```python
from build123d import *

# Parameters (mm, degrees)
BOSS_EXTRU_3_DEPTH = 50
ESQUISSE3_W        = 80
ESQUISSE3_H        = 10
BOSS_EXTRU_4_DEPTH = 50
ESQUISSE4_R        = 15
ESQUISSE4_R_2      = 12
BOSS_EXTRU_5_DEPTH = 5
CONG_1_R           = 2
BOSS_EXTRU_6_DEPTH = 25
BOSS_EXTRU_7_DEPTH = 10


with BuildPart() as part:
    # Esquisse2 → Boss.-Extru.3 (new body)
    with BuildSketch(Plane.XY):
        Polygon((0, 0), (100, 0), (90, 10), (10, 10), align=None)
    extrude(amount=BOSS_EXTRU_3_DEPTH)

    # Esquisse3 → Boss.-Extru.4 (add)
    with BuildSketch(Plane.XY.offset(50)):
        with Locations((50, 15)):
            Rectangle(ESQUISSE3_W, ESQUISSE3_H)
    extrude(amount=-BOSS_EXTRU_4_DEPTH)

    # Esquisse4 → Boss.-Extru.5 (add)
    with BuildSketch(Plane(origin=(0, 20, 0), x_dir=(1, 0, 0), z_dir=(0, 1, 0))):
        with Locations((65, -25)):
            Circle(ESQUISSE4_R)
        with Locations((65, -25)):
            Circle(ESQUISSE4_R_2, mode=Mode.SUBTRACT)
    extrude(amount=BOSS_EXTRU_5_DEPTH)

    # Congé1
    cong_1_edges = [part.edges().sort_by_distance(p)[0] for p in [
        (50, 20, 25),
    ]]
    fillet(cong_1_edges, radius=CONG_1_R)

    # Esquisse5 → Boss.-Extru.6 (add)
    with BuildSketch(Plane(origin=(0, 20, 0), x_dir=(1, 0, 0), z_dir=(0, 1, 0))):
        Polygon((20, 0), (10, 0), (10, -50), (20, -50), (20, -10), (50, -10), (50, 0), align=None)
    extrude(amount=BOSS_EXTRU_6_DEPTH)

    # Esquisse6 → Boss.-Extru.7 (add)
    with BuildSketch(Plane.XY.offset(50)):
        Polygon((20, 45), (50, 20), (20, 20), align=None)
    extrude(amount=-BOSS_EXTRU_7_DEPTH)


solid = part.part
```
Source: CAD feature listing. Evaluate the final solid. Frame: model axes, mm. A direction names the side the tool comes from. Coordinates: 2 decimals unless noted, no trailing zeros. Write each loop counter-clockwise with the first axis right and the second up, starting at its lowest first coordinate (ties: lowest second). Pieces come first, ordered by that corner, then holes. Notation, with made-up numbers: (-35.75, 21) -> (10.25, 21) arc R26 ccw to (10.25, 43) -> close; hole circle Ø2 at (83, 65.5). An arc over 180 degrees is marked (long way). Return JSON: item names as keys, results as strings. Group by question number.
1) Contact query for flat-ended pins moving along their axis: P1, Ø3, axis at y = 16.5, z = 24, coming from the +X side; P2, Ø1.5, axis at y = 17, z = 14.5, coming from the -X side; P3, Ø12, axis at y = 13, z = 12.5, coming from the -X side. Output: stop coordinate, or through.
2) Section query D-D, the plane y = 28.5. Return loops of the section in (x, z).
3) Section query B-B, the plane x = 65. Return loops of the section in (y, z), plus the area to 3 significant figures.
4) Ray query, line 1 along X through (y, z) = (23.65, 25); line 2 along Z through (x, y) = (65, 22); line 3 along Z through (x, y) = (42.5, 32.5). Return the intervals inside material, ascending.
5) Set-up query: faces 1 (the face through (53, 23, 34)), 2 (the face through (40, 17, 0)), 3 (the face through (49, 0, 25)), 4 (the face through (10, 27, 25)), 5 (the face through (90, 15, 25)). Return all of +Z, -Z, +X, -X, +Y, -Y with unobstructed straight access to the full face (end or side cutting, diameter ignored); none if empty.
6) Mould query, pull axis Z, two halves, no side actions, for faces 6 (the face through (56.156, 22.465, 16.89)), 7 (the face through (35, 32, 10)), 8 (the face through (58, 25, 15)), 9 (the face through (40, 18, 50)). Classes: +Z half, -Z half, draft (parallel to the pull), parting line (faces both ways), or undercut.
7) Section query A-A, the plane z = 25. Return loops of the section in (x, y), plus the area to 3 significant figures.
8) Section query C-C, the plane y = 34. Return loops of the section in (x, z).
From the geometry:
{
 "1": {"P1": "x = 90", "P2": "x = 10", "P3": "x = 7"},
 "2": {"outline": "(10, 0) -> (50, 0) -> (50, 10) -> (20, 10) -> (20, 40) -> (39.8, 40) -> (39.8, 50) -> (10, 50) -> close"},
 "3": {"outline": "(0, 0) -> (20, 0) -> (20, 8) arc R2 cw to (22, 10) -> (25, 10) -> (25, 13) -> (20, 13) -> (20, 37) -> (25, 37) -> (25, 40) -> (22, 40) arc R2 cw to (20, 42) -> (20, 50) -> (0, 50) -> close", "area": "1,030 mm²"},
 "4": {"line 1": "10 to 20, 50 to 53, 77 to 80", "line 2": "10 to 13, 37 to 40", "line 3": "0 to 10"},
 "5": {"face 1": "+Y", "face 2": "-Z, +X, -X, +Y, -Y", "face 3": "+Z, -Z, +X, -X, -Y", "face 4": "+Z, -Z, -X, +Y", "face 5": "+Z, -Z, +X, +Y"},
 "6": {"face 6": "undercut", "face 7": "undercut", "face 8": "draft", "face 9": "+Z half"},
 "7": {"outline": "(0, 0) -> (100, 0) -> (90, 10) -> (90, 20) -> (82, 20) arc R2 cw to (80, 22) -> (80, 25) -> (77, 25) -> (77, 20) -> (53, 20) -> (53, 25) -> (50, 25) -> (50, 22) arc R2 cw to (48, 20) -> (20, 20) -> (20, 45) -> (10, 45) -> (10, 10) -> close", "area": "1,980 mm²"},
 "8": {"outline": "(10, 0) -> (50, 0) -> (50, 10) -> (20, 10) -> (20, 40) -> (33.2, 40) -> (33.2, 50) -> (10, 50) -> close"}
}
